from build123d import *

# Parameters (mm, degrees)
CYLINDER002_R            = 41
CYLINDER002_DEPTH        = 10
CYLINDER001_R            = 45.5
CYLINDER001_DEPTH        = 10
CYLINDER004_R            = 46.5
CYLINDER004_DEPTH        = 2
BOX002_W                 = 50
BOX002_H                 = 9
BOX002_DEPTH             = 2
FILLET_R                 = 4
CYLINDER003_R            = 2
CYLINDER003_DEPTH        = 10
ARRAY_X_COUNT            = 2
ARRAY_X_PITCH            = 65
ARRAY_Y_COUNT            = 2
ARRAY_Y_PITCH            = 10
BOX001_W                 = 4
BOX001_H                 = 10
BOX001_DEPTH             = 10
ARRAY001_X_COUNT         = 2
ARRAY001_X_PITCH         = 65
BOX_W                    = 83
BOX_H                    = 50
BOX_DEPTH                = 2
FILLET001_R              = 4
FILLET004_R              = 2
CYLINDER_W               = 46.5
CYLINDER_H               = 6
CYLINDER_ANGLE           = 45
FILLET003_R              = 3
ARRAY002_COUNT           = 4
ARRAY002_PLACEMENT_ANGLE = 22.5


with BuildPart() as hole_cylinder:
    # Cylinder002 → Cylinder002 (new body)
    with BuildSketch(Plane.XY):
        Circle(CYLINDER002_R)
    extrude(amount=CYLINDER002_DEPTH)


with BuildPart() as extract_fusion:
    # Cylinder001 → Cylinder001 (new body)
    with BuildSketch(Plane.XY.offset(2)):
        Circle(CYLINDER001_R)
    extrude(amount=CYLINDER001_DEPTH)

    # Fusion001: union hole cylinder
    add(hole_cylinder.part)


with BuildPart() as outer_cylinder:
    # Cylinder004 → Cylinder004 (new body)
    with BuildSketch(Plane.XY):
        Circle(CYLINDER004_R)
    extrude(amount=CYLINDER004_DEPTH)


with BuildPart() as fillet_body:
    # Box002 → Box002 (new body)
    with BuildSketch(Plane(origin=(-25, -58, 0), x_dir=(1, 0, 0), z_dir=(0, 0, 1))):
        with Locations((25, 4.5)):
            Rectangle(BOX002_W, BOX002_H)
    extrude(amount=BOX002_DEPTH)

    # Fillet
    fillet_edges = [fillet_body.edges().sort_by_distance(p)[0] for p in [
        (-25, -49, 1),
        (25, -49, 1),
    ]]
    fillet(fillet_edges, radius=FILLET_R)


with BuildPart() as hole_array:
    # Cylinder003 → Cylinder003 (new body)
    with BuildSketch(Plane.XY):
        Circle(CYLINDER003_R)
    extrude(amount=CYLINDER003_DEPTH)

    # Array X: hole array ×2


with BuildPart() as hole_array_1:
    add(hole_array.part)
    with Locations(*[(i * ARRAY_X_PITCH, 0, 0) for i in range(1, ARRAY_X_COUNT)]):
        add(hole_array.part)

    # Array Y: hole array ×2


with BuildPart() as hole_array_2:
    add(hole_array_1.part)
    with Locations(*[(0, i * ARRAY_Y_PITCH, 0) for i in range(1, ARRAY_Y_COUNT)]):
        add(hole_array_1.part)


with BuildPart() as fusion003:
    # Box001 → Box001 (new body)
    with BuildSketch(Plane(origin=(-2, 0, 0), x_dir=(1, 0, 0), z_dir=(0, 0, 1))):
        with Locations((2, 5)):
            Rectangle(BOX001_W, BOX001_H)
    extrude(amount=BOX001_DEPTH)

    # Array001 X: Fusion003 ×2


with BuildPart() as fusion003_1:
    add(fusion003.part)
    with Locations(*[(i * ARRAY001_X_PITCH, 0, 0) for i in range(1, ARRAY001_X_COUNT)]):
        add(fusion003.part)

    # Fusion002: union hole array
    add(hole_array_2.part)


with BuildPart() as fusion003_2:
    # Fusion002 placement: moved
    add(fusion003_1.part.moved(Location((-32, -62, 0))))

    # Fusion003: union Fillet body
    add(fillet_body.part)


with BuildPart() as fillet004:
    # Box → Box (new body)
    with BuildSketch(Plane(origin=(-41, -58, 0), x_dir=(1, 0, 0), z_dir=(0, 0, 1))):
        with Locations((41.5, 25)):
            Rectangle(BOX_W, BOX_H)
    extrude(amount=BOX_DEPTH)

    # Fillet001
    fillet001_edges = [fillet004.edges().sort_by_distance(p)[0] for p in [
        (-41, -58, 1),
        (42, -58, 1),
    ]]
    fillet(fillet001_edges, radius=FILLET001_R)

    # Cut001: cut Fusion003
    add(fusion003_2.part, mode=Mode.SUBTRACT)

    # Fillet004
    fillet004_edges = [fillet004.edges().sort_by_distance(p)[0] for p in [
        (35, -58, 1),
        (31, -58, 1),
        (25, -58, 1),
        (-25, -58, 1),
        (-30, -58, 1),
        (-34, -58, 1),
    ]]
    fillet(fillet004_edges, radius=FILLET004_R)


with BuildPart() as obj1:
    # Cylinder → Cylinder (revolve)
    with BuildSketch(Plane.XZ):
        with Locations((23.25, 3)):
            Rectangle(CYLINDER_W, CYLINDER_H)
    revolve(axis=Axis((0, 0, 0), (0, 0, 1)), revolution_arc=CYLINDER_ANGLE)

    # Fillet003
    fillet003_edges = [obj1.edges().sort_by_distance(p)[0] for p in [
        (23.25, 0, 6),
        (16.440233, 16.440233, 6),
    ]]
    fillet(fillet003_edges, radius=FILLET003_R)

    # Array002: obj1 ×4 about axis
    array002_axis = Axis((0, 0, 0), (0, 0, 1))


with BuildPart() as obj1_1:
    add(obj1.part)
    for i in range(1, ARRAY002_COUNT):
        add(obj1.part.rotate(array002_axis, i * 360 / ARRAY002_COUNT))


with BuildPart() as obj1_2:
    # Array002 placement: moved
    add(obj1_1.part.rotate(Axis((0, 0, 0), (0, 0, 1)), ARRAY002_PLACEMENT_ANGLE))

    # Fusion: union outer cylinder, Fillet004
    add(outer_cylinder.part)
    add(fillet004.part)

    # Cut: cut extract fusion
    add(extract_fusion.part, mode=Mode.SUBTRACT)


solid = obj1_2.part
The listing builds one solid part. Answer for the finished solid, in the listing's coordinates (mm). A direction names the side the tool comes from. Coordinates: 2 decimals unless noted, no trailing zeros. Loops run counter-clockwise (first coordinate to the right, second up) from the corner with the lowest first, then second, coordinate; pieces in that order, holes last. Notation, with made-up numbers: M 2.5,-29 L 7.5,-29 A10 cw 7.5,-22 Z; hole C -11,63 d7. An arc over 180 degrees is marked long. Answer in a Markdown table with one row per item.
1) Find the intervals of material crossed by probe 1 along Y at (x, z) = (0, 1.45); probe 2 along Y at (x, z) = (38.5, 3.75); probe 3 along Z at (x, y) = (42, 1.5), in increasing order.
Answers below:
| item | result |
|---|---|
| probe 1 | -49 to -41, 41 to 46.5 |
| probe 2 | -26.08 to -24.25, 24.25 to 26.08 |
| probe 3 | 0 to 2 |
2) Find section B-B (y = 33). Determine the outline of the cut face in (x, z).
Answers below:
| item | result |
|---|---|
| outline | M -32.76,0 L -24.33,0 L -24.33,2 L -31.32,2 L -31.32,6 L -32.76,6 Z; M 24.33,0 L 32.76,0 L 32.76,6 L 31.32,6 L 31.32,2 L 24.33,2 Z |
3) Find section C-C (x = 5). Determine the outline of the cut face in (y, z).
Answers below:
| item | result |
|---|---|
| outline | M -49,0 L -40.69,0 L -40.69,2 L -49,2 Z; M 40.69,0 L 46.23,0 L 46.23,2 L 40.69,2 Z |
4) Which of the six approach directions +Z, -Z, +X, -X, +Y, -Y give full straight-line access (tool end or side, diameter ignored) to faces 1 (the cylindrical face through (-23.859, -50.203, 1.014)), 2 (the cylindrical face through (32.35, 31.996, 3.972)), 3 (the cylindrical face through (-18.421, 42.115, 5.145))?
Answers below:
| item | result |
|---|---|
| face 1 | +Z, -Z, -Y |
| face 2 | +Z |
| face 3 | +Z, +Y |
5) Given pin 1 (2 mm diameter, centred on y = -39.5, z = 1.5, fed in from -X); pin 2 (3 mm diameter, centred on x = -5.5, z = 5, fed in from +Y); pin 3 (1 mm diameter, centred on x = -12.5, z = 1.5, fed in from +Y); pin 4 (1 mm diameter, centred on y = -53.5, z = 1.5, fed in from +X), each flat-ended and moving along its own axis, determine where each tip first touches the part or whether it passes through.
Answers below:
| item | result |
|---|---|
| pin 1 | x = -41 |
| pin 2 | through |
| pin 3 | y = 44.92 |
| pin 4 | x = 42 |
6) Find section A-A (x = -8.5). Determine the outline of the cut face in (y, z).
Answers below:
| item | result |
|---|---|
| outline | M -49,0 L -40.11,0 L -40.11,2 L -49,2 Z; M 40.11,0 L 45.72,0 L 45.72,2 L 40.11,2 Z |
